Here's the drawing with two shaded views (mm, measured from the low corner). I have some questions. A direction names the side the tool comes from. Round coordinates to 2 decimals unless told otherwise and drop trailing zeros. Order: outer loops, then holes, each group sorted by start corner. A loop starts at its lowest first (then second) coordinate and runs counter-clockwise, first axis right, second up. Notation, with made-up numbers: (36, 29.5) -> (77, 29.5) arc R8 cw to (77, 41.5) -> close; hole circle Ø6 at (35, 83). An arc over 180 degrees is marked (long way). Answer in a Markdown table with one row per item.
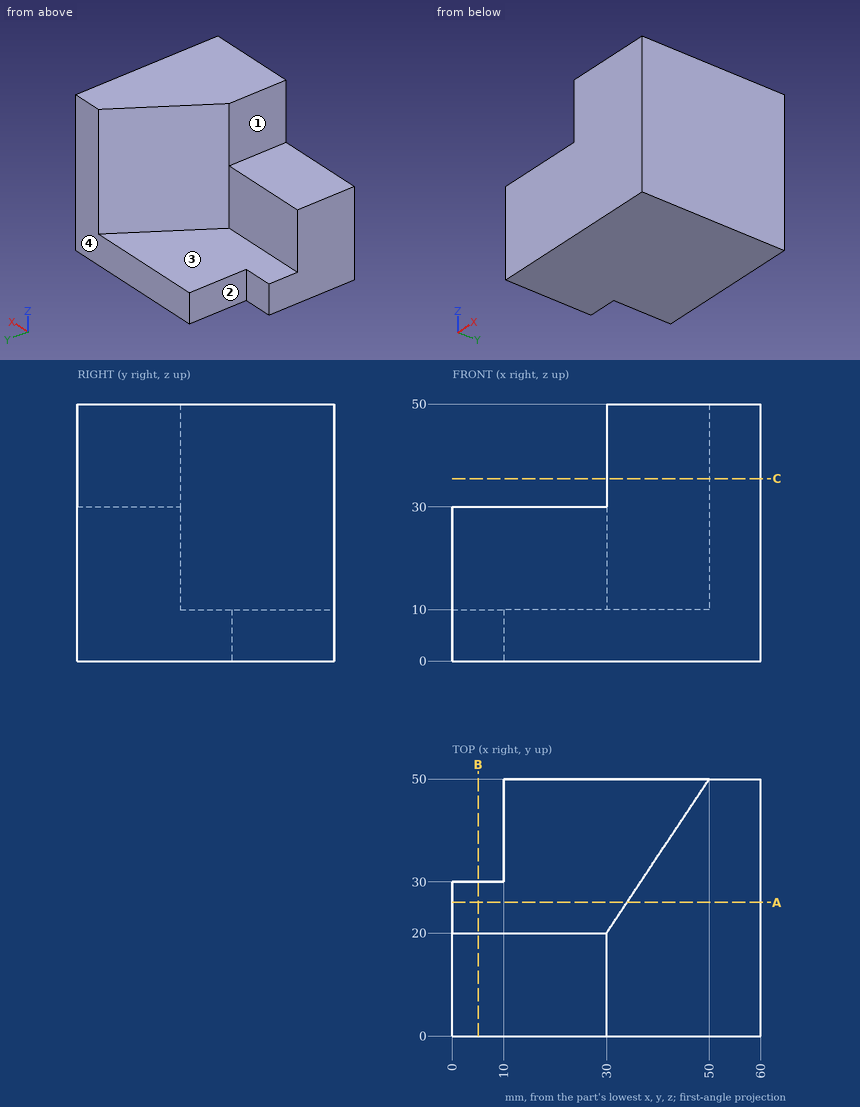
1. For the marked faces 1, 2, 3 and 4, which set-ups out of +Z, -Z, +X, -X, +Y, -Y let a thin tool reach every point of the face, with its end or its side?
Numbers:
| item | result |
|---|---|
| face 1 | +Z, -X, +Y, -Y |
| face 2 | +Z, -Z, -X, +Y |
| face 3 | +Z, -X, +Y |
| face 4 | +Z, -Z, +X, -X, +Y |
2. Suppose I cut it at C-C on z = 35.5. Write out the boundary of the cut face in (x, y), then the cut area to 3 significant figures.
Numbers:
| item | result |
|---|---|
| outline | (30, 0) -> (60, 0) -> (60, 50) -> (50, 50) -> (30, 20) -> close |
| area | 1,200 mm2 |
3. Please list where these lines run through material, in increasing order: line 1 along X through (y, z) = (3, 42.5); line 2 along Z through (x, y) = (20.5, 9); line 3 along Z through (x, y) = (7, 24.5).
Numbers:
| item | result |
|---|---|
| line 1 | x = 30 to 60 |
| line 2 | z = 0 to 30 |
| line 3 | z = 0 to 10 |
4. Suppose I cut it at B-B on x = 5. Write out the boundary of the cut face in (y, z).
Numbers:
| item | result |
|---|---|
| outline | (0, 0) -> (30, 0) -> (30, 10) -> (20, 10) -> (20, 30) -> (0, 30) -> close |
5. Suppose I cut it at A-A on y = 26. Write out the boundary of the cut face in (x, z).
Numbers:
| item | result |
|---|---|
| outline | (0, 0) -> (60, 0) -> (60, 50) -> (34, 50) -> (34, 10) -> (0, 10) -> close |
6. For pin 1 Ø4 at (x, z) = (52.5, 37) entering from -Y; pin 2 Ø16 at (x, y) = (17, 5.5) entering from +Z; pin 3 Ø11 at (y, z) = (40.5, 4.5) entering from -X; pin 4 Ø22 at (x, z) = (20.5, 24) entering from +Y, each with a flat end and sliding along its axis, tell me the tip position at first contact or that it passes through.
Numbers:
| item | result |
|---|---|
| pin 1 | stops at y = 0 |
| pin 2 | stops at z = 30 |
| pin 3 | stops at x = 10 |
| pin 4 | stops at y = 22.25 |
